Geometry check sheet. Reference: the model listing, model coordinates, mm. A direction names the side the tool comes from. Coordinates: 2 decimals unless noted, no trailing zeros. Loops run counter-clockwise (first coordinate to the right, second up) from the corner with the lowest first, then second, coordinate; pieces in that order, holes last. Notation, with made-up numbers: (-12.75, 5) - (13.25, 5) arc R16 ccw to (13.25, 9) - close; hole circle Ø4 at (-5, 83). An arc over 180 degrees is marked (long way). Write each question's results on one line, items separated by ' | '. Start each with the question number.
(1) Access from +Z, -Z, +X, -X, +Y, -Y to the whole of each face (thin tool, end or side, straight path). Record for faces 4 (the face through (51, 0.7, 29.4)), 5 (the face through (51, 5.3, 29.4)), 6 (the face through (18, 3, 5)), 7 (the face through (12, 3, 5)).
(2) Sectioned sample at B-B (y = 4). Enter the section's corners in (x, z), plus the area to 3 significant figures.
(3) Sectioned sample at D-D (z = 21.5). Enter the section's corners in (x, y).
(4) Sectioned sample at A-A (z = 4.25). Enter the section's corners in (x, y).
(5) Mould release check, pull along X, two halves, no side actions. Record for faces 1 (the face through (45, 3, 5)), 2 (the face through (71, 3, 27)), 3 (the face through (25, 3, 16)): pulls with the +X half, pulls with the -X half, needs draft (parallel to the pull), parting line crosses it, or undercut.
(6) Sectioned sample at C-C (x = 25). Enter the section's corners in (y, z).
(7) Material ranges on probe 1 along X at (y, z) = (4.25, 7); probe 2 along Z at (x, y) = (29, 2.25); probe 3 along X at (y, z) = (5.75, 19.25), recorded low to high.
(8) Go/stop test with flat-tipped pins: pin 1 Ø3 at (x, y) = (27, 3.5) entering from -Z; pin 2 Ø1.5 at (y, z) = (4.5, 7) entering from -X; pin 3 Ø10 at (x, z) = (13, 20) entering from +Y; pin 4 Ø1.5 at (y, z) = (4.5, 12) entering from +X. Record where each tip stops, or that it passes through.
from build123d import *

# Parameters (mm, degrees)
RESSALTO_EXTRUS_O3_DEPTH = 6
CORTE_EXTRUS_O1_DEPTH    = 20


with BuildPart() as part:
    # Esboço1 → Ressalto-extrusão3 (new body)
    with BuildSketch(Plane(origin=(0, 0, 0), x_dir=(1, 0, 0), z_dir=(0, 1, 0))):
        Polygon((12, -10), (6, -10), (6, -16), (45, -16), (45, -30), (71, -30), (71, -24), (51, -24), (51, 0), (45, 0), (45, -10), (18, -10), (18, 0), (12, 0), align=None)
    extrude(amount=RESSALTO_EXTRUS_O3_DEPTH)

    # Esboço2 → Corte-extrusão1 (cut)
    with BuildSketch(Plane(origin=(71, 0, 0), x_dir=(0, 0, -1), z_dir=(1, 0, 0))):
        with BuildLine():
            Line((-30, 6), (-30, 3))
            ThreePointArc((-30, 3), (-29.121320344, 5.121320344), (-27, 6))
            Line((-27, 6), (-30, 6))
        make_face()
        with BuildLine():
            Line((-24, 6), (-27, 6))
            ThreePointArc((-27, 6), (-24.878679656, 5.121320344), (-24, 3))
            Line((-24, 3), (-24, 6))
        make_face()
        with BuildLine():
            ThreePointArc((-24, 3), (-24.878679656, 0.878679656), (-27, 0))
            Line((-27, 0), (-24, 0))
            Line((-24, 0), (-24, 3))
        make_face()
        with BuildLine():
            ThreePointArc((-27, 0), (-29.121320344, 0.878679656), (-30, 3))
            Line((-30, 3), (-30, 0))
            Line((-30, 0), (-27, 0))
        make_face()
    extrude(amount=-CORTE_EXTRUS_O1_DEPTH, mode=Mode.SUBTRACT)


solid = part.part
Outcome:
1) face 4: +Z, +X, -Y | face 5: +Z, +X, +Y | face 6: -Z, +Y, -Y | face 7: -Z, -X, +Y, -Y
2) outline: (6, 10) - (12, 10) - (12, 0) - (18, 0) - (18, 10) - (45, 10) - (45, 0) - (51, 0) - (51, 24.17) - (71, 24.17) - (71, 29.83) - (51, 29.83) - (51, 30) - (45, 30) - (45, 16) - (6, 16) - close | area: 587 mm2
3) outline: (45, 0) - (51, 0) - (51, 6) - (45, 6) - close
4) outline: (12, 0) - (18, 0) - (18, 6) - (12, 6) - close; (45, 0) - (51, 0) - (51, 6) - (45, 6) - close
5) face 1: undercut | face 2: pulls with the +X half | face 3: needs draft
6) outline: (0, 10) - (6, 10) - (6, 16) - (0, 16) - close
7) probe 1: x = 12 to 18, 45 to 51 | probe 2: z = 10 to 16 | probe 3: x = 45 to 51
8) pin 1: stops at z = 10 | pin 2: stops at x = 12 | pin 3: stops at y = 6 | pin 4: stops at x = 51
